```python
from build123d import *

# Parameters (mm, degrees)
SKETCH1_R           = 1.75
SKETCH1_W           = 5
SKETCH1_H           = 5
SKETCH1_W_2         = 10
BOSS_EXTRUDE1_DEPTH = 5
SKETCH2_R           = 3
CUT_EXTRUDE1_DEPTH  = 3


with BuildPart() as part:
    # Sketch1 → Boss-Extrude1 (new body)
    # profile 1 of 4: a face of its own
    with BuildSketch(Plane(origin=(0, 0, 0), x_dir=(1, 0, 0), z_dir=(0, 1, 0))):
        Polygon((-21.909620991, 19.482507289), (-21.909620991, -11.767492711), (23.090379009, -11.767492711), (23.090379009, 19.482507289), (-6.909620991, 19.482507289), (-16.909620991, 19.482507289), align=None)
        with Locations(Location((0.590379009, 8.532507289, 0), (0, 0, 270))):
            Circle(SKETCH1_R, mode=Mode.SUBTRACT)
        with Locations((15.590379009, 8.732507289)):
            Rectangle(SKETCH1_W, SKETCH1_H, mode=Mode.SUBTRACT)
    # profile 2 of 4: a face of its own
    with BuildSketch(Plane(origin=(0, 0, 0), x_dir=(1, 0, 0), z_dir=(0, 1, 0))):
        Polygon((23.090379009, -11.767492711), (-21.909620991, -11.767492711), (-21.909620991, -43.017492711), (-16.909620991, -43.017492711), (-6.909620991, -43.017492711), (23.090379009, -43.017492711), align=None)
        with Locations(Location((0.590379009, -32.067492711, 0), (0, 0, 270))):
            Circle(SKETCH1_R, mode=Mode.SUBTRACT)
        with Locations((15.590379009, -32.267492711)):
            Rectangle(SKETCH1_W, SKETCH1_H, mode=Mode.SUBTRACT)
    # profile 3 of 4: a face of its own
    with BuildSketch(Plane(origin=(0, 0, 0), x_dir=(1, 0, 0), z_dir=(0, 1, 0))):
        with Locations((-11.909620991, -45.517492711)):
            Rectangle(SKETCH1_W_2, SKETCH1_H)
    # profile 4 of 4: a face of its own
    with BuildSketch(Plane(origin=(0, 0, 0), x_dir=(1, 0, 0), z_dir=(0, 1, 0))):
        with Locations((-11.909620991, 21.982507289)):
            Rectangle(SKETCH1_W_2, SKETCH1_H)
    extrude(amount=BOSS_EXTRUDE1_DEPTH)

    # Sketch2 → Cut-Extrude1 (cut)
    with BuildSketch(Plane(origin=(0, 5, 0), x_dir=(1, 0, 0), z_dir=(0, 1, 0))):
        with Locations(Location((0.590379009, -32.067492711, 0), (0, 0, 270))):
            Circle(SKETCH2_R)
        with Locations(Location((0.590379009, 8.532507289, 0), (0, 0, 270))):
            Circle(SKETCH2_R)
    extrude(amount=-CUT_EXTRUDE1_DEPTH, mode=Mode.SUBTRACT)


solid = part.part
```
The listing builds one solid part. Answer for the finished solid, in the listing's coordinates (mm). A direction names the side the tool comes from. Give positions to 0.01 mm unless a question says otherwise; leave off trailing zeros. Loops run counter-clockwise (first coordinate to the right, second up) from the corner with the lowest first, then second, coordinate; pieces in that order, holes last. Notation, with made-up numbers: M 13.5,86 L 22.5,86 A24 cw 22.5,99 Z; hole C -29.5,-19 d4. An arc over 180 degrees is marked long. One line per item, written item: value.
1. Section A-A on x = 17 is taken. Determine the outline of the cut face in (y, z), plus the area to 4 significant figures.
Found:
outline: M 0,-19.48 L 5,-19.48 L 5,-11.23 L 0,-11.23 Z; M 0,-6.23 L 5,-6.23 L 5,29.77 L 0,29.77 Z; M 0,34.77 L 5,34.77 L 5,43.02 L 0,43.02 Z
area: 262.5 mm^2
2. Section C-C on x = -18 is taken. Determine the outline of the cut face in (y, z).
Found:
outline: M 0,-19.48 L 5,-19.48 L 5,43.02 L 0,43.02 Z
3. Section B-B on y = 2.8 is taken. Determine the outline of the cut face in (x, z), plus the area to 3 significant figures.
Found:
outline: M -21.91,-19.48 L -16.91,-19.48 L -16.91,-24.48 L -6.91,-24.48 L -6.91,-19.48 L 23.09,-19.48 L 23.09,43.02 L -6.91,43.02 L -6.91,48.02 L -16.91,48.02 L -16.91,43.02 L -21.91,43.02 Z; hole C 0.59,-8.53 d6; hole C 0.59,32.07 d6; hole M 13.09,-11.23 L 18.09,-11.23 L 18.09,-6.23 L 13.09,-6.23 Z; hole M 13.09,29.77 L 18.09,29.77 L 18.09,34.77 L 13.09,34.77 Z
area: 2,810 mm^2
4. Each of these flat-tipped pins is pushed along its axis until it touches: P1, Ø2, axis at x = 11, y = 2.5, coming from the +Z side; P2, Ø1.8, axis at x = 1.5, z = 33, coming from the +Y side; P3, Ø4, axis at x = 0.59, z = 32.07, coming from the -Y side; P4, Ø2, axis at x = 5.5, y = 3.5, coming from the -Z side. Where does it stop, or does it pass through?
Found:
P1: z = 43.02
P2: y = 2
P3: y = 0
P4: z = -19.48
5. For faces 4 (the face through (3.565, 3.521, -8.923)), 5 (the face through (-6.91, 2, 46)), 6 (the face through (18.09, 2, -9)), determine the directions among +Z, -Z, +X, -X, +Y, -Y from which every point of the face is accessible in a straight line to the end or side of a thin tool.
Found:
face 4: +Y
face 5: +Z, +X, +Y, -Y
face 6: +Y, -Y
6. Find the intervals of material crossed by probe 1 along Z at (x, y) = (15, 0.65); probe 2 along Z at (x, y) = (0, 3.45); probe 3 along Z at (x, y) = (-5.5, 0.7), in increasing order.
Found:
probe 1: -19.48 to -11.23, -6.23 to 29.77, 34.77 to 43.02
probe 2: -19.48 to -11.47, -5.59 to 29.13, 35.01 to 43.02
probe 3: -19.48 to 43.02
7. For a pull along X with two mould halves and no side action, classify faces 1 (the face through (-21.91, 2, 11)), 2 (the face through (-19, 2, -19.483)), 3 (the face through (16, 2, -11.233)) as pulls with the +X half, pulls with the -X half, needs draft (parallel to the pull), parting line crosses it, or undercut.
Found:
face 1: pulls with the -X half
face 2: needs draft
face 3: undercut
